from build123d import *

# Parameters (mm, degrees)
BOSS_EXTRUDE1_DEPTH                = 60
SKETCH2_W                          = 15
SKETCH2_H                          = 20
CUT_EXTRUDE1_DEPTH                 = 85.888209544
CUT_EXTRUDE2_REACH                 = 85.66
SKETCH4_W                          = 2.5
SKETCH4_H                          = 20
CUT_EXTRUDE3_REACH                 = 85.66
SKETCH6_W                          = 2.5
SKETCH6_H                          = 20
CUT_EXTRUDE4_DEPTH                 = 98.632993582
CUT_EXTRUDE5_DEPTH                 = 95.486300493
CUT_EXTRUDE6_DEPTH                 = 85.888209544
F_4_3_4_3_DIAMETER_HOLE1_D         = 4.3
F_4_3_4_3_DIAMETER_HOLE1_DEPTH     = 75.600067507
F_4_3_4_3_DIAMETER_HOLE2_D         = 4.3
F_4_3_4_3_DIAMETER_HOLE2_DEPTH     = 75.600067507
F_4_3_4_3_DIAMETER_HOLE3_D         = 4.3
F_4_3_4_3_DIAMETER_HOLE3_DEPTH     = 4.11
F_25_0_START                       = -17.38342993
F_25_0_25_DIAMETER_HOLE1_DEPTH     = 16.551366025
F_4_3_4_3_DIAMETER_HOLE4_D         = 4.3
F_4_3_4_3_DIAMETER_HOLE4_DEPTH     = 4.11
F_25_0_START_2                     = 0.832063905
F_25_0_25_DIAMETER_HOLE2_OUTLINE_R = 12.5
F_25_0_25_DIAMETER_HOLE2_DEPTH     = 16.551366025
F_23_0_23_DIAMETER_HOLE1_D         = 23
F_23_0_23_DIAMETER_HOLE1_DEPTH     = 4.22
F_3_3_3_3_DIAMETER_HOLE1_D         = 3.3
F_3_3_3_3_DIAMETER_HOLE1_DEPTH     = 4.22
M3_5_CLEARANCE_HOLE1_D             = 3.85
FILLET1_R                          = 3
FILLET2_R                          = 4.5


# Read off the part's stored shape, not the designer's step: Ø25.0 (25) Diameter Hole1, Ø25.0 (25) Diameter Hole2
with BuildPart() as part:
    # Sketch1 → Boss-Extrude1 (new body)
    with BuildSketch(Plane.XZ):
        with BuildLine():
            Line((32.375, -18.691714965), (15.054491924, -8.691714965))
            Line((15.054491924, -8.691714965), (43.054491924, 39.805707647))
            Line((43.054491924, 39.805707647), (39.495127515, 41.860707647))
            Line((39.495127515, 41.860707647), (28.69628865, 23.15657007))
            Line((28.69628865, 23.15657007), (-28.69628865, 23.15657007))
            Line((-28.69628865, 23.15657007), (-39.495127515, 41.860707647))
            Line((-39.495127515, 41.860707647), (-43.054491924, 39.805707647))
            Line((-43.054491924, 39.805707647), (-15.054491924, -8.691714965))
            Line((-15.054491924, -8.691714965), (-32.375, -18.691714965))
            ThreePointArc((-32.375, -18.691714965), (0, -37.38342993), (32.375, -18.691714965))
        make_face()
    extrude(amount=-BOSS_EXTRUDE1_DEPTH)

    # Sketch2 → Cut-Extrude1 (cut, through all)
    with BuildSketch(Plane.XZ):
        with Locations((0, -22.94342993)):
            Rectangle(SKETCH2_W, SKETCH2_H)
    extrude(amount=-CUT_EXTRUDE1_DEPTH, mode=Mode.SUBTRACT)

    # Sketch4 → Cut-Extrude2 (cut, up to next)
    with BuildSketch(Plane.XZ.offset(-1.75), mode=Mode.PRIVATE) as cut_extrude2_sk1:
        with Locations((8.75, -22.94342993)):
            Rectangle(SKETCH4_W, SKETCH4_H)
    cut_extrude2_tool1 = extrude(cut_extrude2_sk1.sketch, amount=-CUT_EXTRUDE2_REACH, mode=Mode.PRIVATE) & part.part
    add(cut_extrude2_tool1.solids().sort_by_distance((8.75, 1.75, -22.94343))[0], mode=Mode.SUBTRACT)

    # Sketch6 → Cut-Extrude3 (cut, up to next)
    with BuildSketch(Plane.XZ.offset(-1.75), mode=Mode.PRIVATE) as cut_extrude3_sk1:
        with Locations((-8.75, -22.94342993)):
            Rectangle(SKETCH6_W, SKETCH6_H)
    cut_extrude3_tool1 = extrude(cut_extrude3_sk1.sketch, amount=-CUT_EXTRUDE3_REACH, mode=Mode.PRIVATE) & part.part
    add(cut_extrude3_tool1.solids().sort_by_distance((-8.75, 1.75, -22.94343))[0], mode=Mode.SUBTRACT)

    # Sketch7 → Cut-Extrude4 (cut, through all)
    with BuildSketch(Plane(origin=(15.054491924, 0, -8.691714965), x_dir=(-0.4999999999999995, 0, -0.866025403784439), z_dir=(0.8660254037844389, 0, -0.49999999999999944))):
        with BuildLine():
            Line((-49, 37.15), (-49, 22.85))
            ThreePointArc((-49, 22.85), (-46.15, 20), (-43.3, 22.85))
            Line((-43.3, 22.85), (-43.3, 37.15))
            ThreePointArc((-43.3, 37.15), (-46.15, 40), (-49, 37.15))
        make_face()
    extrude(amount=-CUT_EXTRUDE4_DEPTH, mode=Mode.SUBTRACT)

    # Sketch8 → Cut-Extrude5 (cut, through all)
    with BuildSketch(Plane(origin=(-11.495127515, 0, -6.636714965), x_dir=(0.5000000000000004, 0, -0.8660254037844385), z_dir=(0.8660254037844384, 0, 0.5000000000000003))):
        with BuildLine():
            Line((-49, 37.15), (-49, 22.85))
            ThreePointArc((-49, 22.85), (-46.15, 20), (-43.3, 22.85))
            Line((-43.3, 22.85), (-43.3, 37.15))
            ThreePointArc((-43.3, 37.15), (-46.15, 40), (-49, 37.15))
        make_face()
    extrude(amount=-CUT_EXTRUDE5_DEPTH, mode=Mode.SUBTRACT)

    # Sketch9 → Cut-Extrude6 (cut, through all)
    with BuildSketch(Plane(origin=(0, 60, 0), x_dir=(-1, 0, 0), z_dir=(0, 1, 0))):
        with BuildLine():
            Line((22.795768899, 18.93657007), (-22.795768899, 18.93657007))
            ThreePointArc((-22.795768899, 18.93657007), (-24.527819706, 17.93657007), (-24.527819706, 15.93657007))
            Line((-24.527819706, 15.93657007), (-10.163345009, -8.94342993))
            Line((-10.163345009, -8.94342993), (10.163345009, -8.94342993))
            Line((10.163345009, -8.94342993), (24.527819706, 15.93657007))
            ThreePointArc((24.527819706, 15.93657007), (24.527819706, 17.93657007), (22.795768899, 18.93657007))
        make_face()
    extrude(amount=-CUT_EXTRUDE6_DEPTH, mode=Mode.SUBTRACT)

    # Ø4.3 (4.3) Diameter Hole1
    with Locations(Plane(origin=(-15.054491924, 0, -8.691714965), x_dir=(-0.5000000000000003, 0, 0.8660254037844385), z_dir=(-0.8660254037844385, 0, -0.5000000000000003))):
        with Locations((46, 9.48944756), (46, 50)):
            Hole(F_4_3_4_3_DIAMETER_HOLE1_D / 2, depth=F_4_3_4_3_DIAMETER_HOLE1_DEPTH)

    # Ø4.3 (4.3) Diameter Hole2
    with Locations(Plane(origin=(15.054491924, 0, -8.691714965), x_dir=(-0.4999999999999995, 0, -0.866025403784439), z_dir=(0.8660254037844389, 0, -0.49999999999999944))):
        with Locations((-46, 9.48944756), (-46, 50)):
            Hole(F_4_3_4_3_DIAMETER_HOLE2_D / 2, depth=F_4_3_4_3_DIAMETER_HOLE2_DEPTH)

    # Ø4.3 (4.3) Diameter Hole3
    with Locations(Plane(origin=(-15.054491924, 0, -8.691714965), x_dir=(-0.5000000000000003, 0, 0.8660254037844385), z_dir=(-0.8660254037844385, 0, -0.5000000000000003))):
        with Locations((8.5, 9.48944756), (8.5, 50)):
            Hole(F_4_3_4_3_DIAMETER_HOLE3_D / 2, depth=F_4_3_4_3_DIAMETER_HOLE3_DEPTH)

    # Ø25.0 (25) Diameter Hole1 outline → Ø25.0 (25) Diameter Hole1 (cut)
    with BuildSketch(Plane(origin=(0, 0, 0), x_dir=(0.5000000000000003, 0, -0.8660254037844385), z_dir=(0.8660254037844385, 0, 0.5000000000000003)).offset(F_25_0_START)):
        with BuildLine():
            ThreePointArc((-22.346459974, 21.168797028), (-1, 30), (-22.346459974, 38.831202972))
            ThreePointArc((-22.346459974, 38.831202972), (-26, 30), (-22.346459974, 21.168797028))
        make_face()
    extrude(amount=F_25_0_25_DIAMETER_HOLE1_DEPTH, mode=Mode.SUBTRACT)

    # Ø4.3 (4.3) Diameter Hole4
    with Locations(Plane(origin=(15.054491924, 0, -8.691714965), x_dir=(-0.4999999999999995, 0, -0.866025403784439), z_dir=(0.8660254037844389, 0, -0.49999999999999944))):
        with Locations((-8.5, 9.48944756), (-8.5, 50)):
            Hole(F_4_3_4_3_DIAMETER_HOLE4_D / 2, depth=F_4_3_4_3_DIAMETER_HOLE4_DEPTH)

    # Ø25.0 (25) Diameter Hole2 outline → Ø25.0 (25) Diameter Hole2 (cut)
    with BuildSketch(Plane(origin=(0, 0, 0), x_dir=(0.49999999999999956, 0, 0.8660254037844389), z_dir=(0.8660254037844388, 0, -0.4999999999999999)).offset(F_25_0_START_2)):
        with Locations((13.5, -30)):
            Circle(F_25_0_25_DIAMETER_HOLE2_OUTLINE_R)
    extrude(amount=F_25_0_25_DIAMETER_HOLE2_DEPTH, mode=Mode.SUBTRACT)

    # Ø23.0 (23) Diameter Hole1
    with Locations(Plane.XY.offset(23.15657007)):
        with Locations((0, 30)):
            Hole(F_23_0_23_DIAMETER_HOLE1_D / 2, depth=F_23_0_23_DIAMETER_HOLE1_DEPTH)

    # Ø3.3 (3.3) Diameter Hole1
    with Locations(Plane.XY.offset(23.15657007)):
        with Locations((15.5, 45.5), (15.5, 14.5), (-15.5, 14.5), (-15.5, 45.5)):
            Hole(F_3_3_3_3_DIAMETER_HOLE1_D / 2, depth=F_3_3_3_3_DIAMETER_HOLE1_DEPTH)

    # M3.5 Clearance Hole1 (through all)
    with Locations(Plane(origin=(0, 0, 0), x_dir=(-1, 0, 0), z_dir=(0, -1, 0))):
        with Locations((-27.375, -20.045794742), (27.375, -20.045794742)):
            Hole(M3_5_CLEARANCE_HOLE1_D / 2)

    # Fillet1
    fillet1_edges = [part.edges().sort_by_distance(p)[0] for p in [
        (-10.163345009, 30, -8.94342993),
        (10.163345009, 30, -8.94342993),
        (-39.495127515, 30, 41.860707647),
        (39.495127515, 30, 41.860707647),
    ]]
    fillet(fillet1_edges, radius=FILLET1_R)

    # Fillet2
    fillet2_edges = [part.edges().sort_by_distance(p)[0] for p in [
        (-28.69628865, 30, 23.15657007),
        (28.69628865, 30, 23.15657007),
    ]]
    fillet(fillet2_edges, radius=FILLET2_R)


solid = part.part
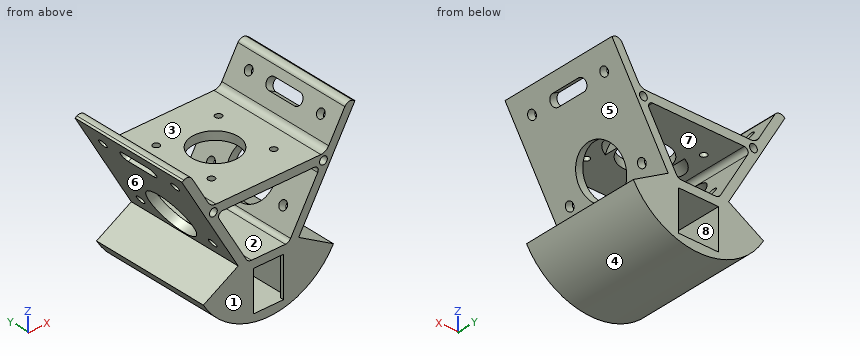
Can you work these out from the model? Positions are in its coordinate system, mm. Face numbers are marked on the shaded views. A direction names the side the tool comes from. Round coordinates to 2 decimals unless told otherwise and drop trailing zeros. Write each loop counter-clockwise with the first axis right and the second up, starting at its lowest first coordinate (ties: lowest second). Pieces come first, ordered by that corner, then holes. Notation, with made-up numbers: M 74.25,23 L 78.25,23 A23 cw 78.25,56 Z; hole C 7.25,62 d6. An arc over 180 degrees is marked long. Use CSV: the item, a comma, the result in double quotes.
(1) Imagine slicing it at B-B (z = 17). Write out the boundary of the cut face in (x, y), plus the area to 3 significant figures.
Check values:
outline,"M -29.89,0 L -24.79,0 L -24.79,60 L -29.89,60 Z; M 24.79,0 L 29.89,0 L 29.89,60 L 24.79,60 Z"
area,"611 mm^2"
(2) I'm going to push flat-ended pins straight in: pin 1 (1 mm diameter, centred on x = 29, y = 20, fed in from -Z); pin 2 (1.2 mm diameter, centred on x = 8, z = -22.5, fed in from +Y); pin 3 (5 mm diameter, centred on y = 19, z = 14.5, fed in from -X). Where does each tip first touch, or does it pass through?
Check values:
pin 1,"z = -24.19"
pin 2,"y = 1.75"
pin 3,"x = -29.89"
(3) Imagine slicing it at A-A (x = 0). Write out the boundary of the cut face in (y, z), plus the area to 3 significant figures.
Check values:
outline,"M 0,-37.38 L 60,-37.38 L 60,-32.94 L 0,-32.94 Z; M 0,-12.94 L 60,-12.94 L 60,-8.94 L 0,-8.94 Z; M 0,18.94 L 18.5,18.94 L 18.5,23.16 L 0,23.16 Z; M 41.5,18.94 L 60,18.94 L 60,23.16 L 41.5,23.16 Z"
area,"663 mm^2"
(4) Imagine slicing it at C-C (y = 30). Count the separate pieces of the cut face and the enclosed holes in it, plus the area to 3 significant figures.
Check values:
separate pieces,"5"
enclosed holes,"3"
area,"1,240 mm^2"
(5) On a 3-axis mill with a long thin cutter (end or side, diameter ignored), from which of +Z, -Z, +X, -X, +Y, -Y can I reach the whole of each face in a straight line? I mean the marked faces 5, 6, 7 and 8. Say none if no direction works.
Check values:
face 5,"+X, +Y, -Y"
face 6,"-X, +Y, -Y"
face 7,"+Y, -Y"
face 8,"+Y"
(6) I need wall thicknesses on line 1 along Y through (x, z) = (0, 21.6); line 2 along Z through (x, y) = (-26.5, 18); line 3 along Z through (x, y) = (-2, 56.5). Which ranges of each line are inside material? Lowest first, please.
Check values:
line 1,"0 to 18.5, 41.5 to 60"
line 2,"-26.37 to -15.3, 11.13 to 18.33, 21.76 to 23.17"
line 3,"-37.33 to -32.94, -12.94 to -8.94, 18.94 to 23.16"
(7) We'd pull the mould along Z, two halves only. Please class the marked faces 1, 2, 3 and 4: +Z half, -Z half, draft (parallel to the pull), parting line (faces both ways), or undercut.
Check values:
face 1,"draft"
face 2,"undercut"
face 3,"+Z half"
face 4,"-Z half"
